Work out the finished part from the listing and answer in its coordinate system (mm). A direction names the side the tool comes from. Coordinates: 2 decimals unless noted, no trailing zeros. Loops run counter-clockwise (first coordinate to the right, second up) from the corner with the lowest first, then second, coordinate; pieces in that order, holes last. Notation, with made-up numbers: (-15.5, 73.25) -> (-6.5, 73.25) arc R17 ccw to (-6.5, 96.25) -> close; hole circle Ø5 at (31.5, 88.25). An arc over 180 degrees is marked (long way). Use a Markdown table: item, result.
from build123d import *


with BuildPart() as part:
    # Sketch1 → Revolve1 (revolve)
    with BuildSketch(Plane.XZ):
        with BuildLine():
            Line((7.540625, 1.6684), (7.540625, 8.725))
            Line((7.540625, 8.725), (7.078744785, 9.525))
            Line((7.078744785, 9.525), (6.35, 9.525))
            Line((6.35, 9.525), (6.35, 0))
            Line((6.35, 0), (11.1125, 0))
            Line((11.1125, 0), (11.1125, 1.1684))
            Line((11.1125, 1.1684), (8.040625, 1.1684))
            ThreePointArc((8.040625, 1.1684), (7.687071609, 1.314846609), (7.540625, 1.6684))
        make_face()
    revolve(axis=Axis((0, 0, 9.525), (0, 0, -1)))


solid = part.part
Q1. For faces 1 (the flat face through (-6, 3, 9.525)), 2 (the flat face through (6, -6, 1.168)), determine the directions among +Z, -Z, +X, -X, +Y, -Y from which every point of the face is accessible in a straight line to the end or side of a thin tool.
Solved:
| item | result |
|---|---|
| face 1 | +Z, +X, -X, +Y, -Y |
| face 2 | +Z |
Q2. Section D-D on y = -8.5 is taken. Determine the outline of the cut face in (x, z).
Solved:
| item | result |
|---|---|
| outline | (-7.16, 0) -> (7.16, 0) -> (7.16, 1.17) -> (-7.16, 1.17) -> close |
Q3. Given pin 1 Ø4 at (x, z) = (-8.5, 8) entering from +Y; pin 2 Ø4 at (x, y) = (-8.5, 8) entering from +Z; pin 3 Ø10 at (x, y) = (0, 0) entering from -Z; pin 4 Ø2 at (y, z) = (3.5, 2) entering from -X, each flat-ended and moving along its own axis, determine where each tip first touches the part or whether it passes through.
Solved:
| item | result |
|---|---|
| pin 1 | y = 3.82 |
| pin 2 | z = 1.17 |
| pin 3 | through |
| pin 4 | x = -10.72 |
Q4. Determine the mould class of faces 3 (the cylindrical face through (-1.38, 6.2, 4.7)), 4 (the cylindrical face through (-7.533, -0.332, 5.246)), 5 (the flat face through (-5, 5, 0)) for opening direction Y: pulls with the +Y half, pulls with the -Y half, needs draft (parallel to the pull), parting line crosses it, or undercut.
Solved:
| item | result |
|---|---|
| face 3 | undercut |
| face 4 | parting line crosses it |
| face 5 | needs draft |
Q5. Section C-C on z = 3.25 is taken. Determine the outline of the cut face in (x, y).
Solved:
| item | result |
|---|---|
| outline | circle Ø15.08 at (0, 0); hole circle Ø12.7 at (0, 0) |
Q6. Consider line 1 (Y direction, x = 0, z = 3.25); line 2 (Z direction, x = 6.75, y = -6.5). Determine where each line is inside the solid, lowest interval first. Write a range as [from, to].
Solved:
| item | result |
|---|---|
| line 1 | [-7.54, -6.35], [6.35, 7.54] |
| line 2 | [0, 1.17] |
